Here's how the part is built. I have some questions about the finished solid (model axes, mm). Face numbers are marked on the shaded views. A direction names the side the tool comes from. Round coordinates to 2 decimals unless told otherwise and drop trailing zeros. Loops run counter-clockwise (first coordinate to the right, second up) from the corner with the lowest first, then second, coordinate; pieces in that order, holes last. Notation, with made-up numbers: M 79.5,-4.5 L 131.5,-4.5 A7 cw 131.5,8.5 Z; hole C 86.5,-16.75 d6. An arc over 180 degrees is marked long. Answer as a JSON object with one key per item and string values.
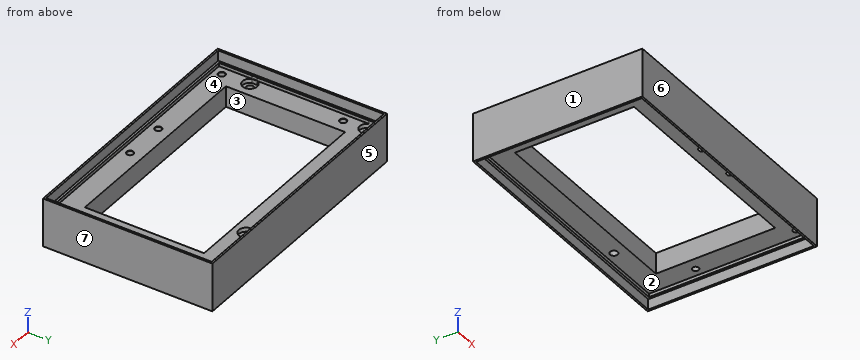
from build123d import *

# Parameters (mm, degrees)
F0_W            = 124.8
F0_H            = 81
F1_DEPTH        = 23.2
F2_W            = 123
F2_H            = 79.2
F3_DEPTH        = 5
F4_W            = 123
F4_H            = 79.2
F5_DEPTH        = 5
F6_W            = 120.8
F6_H            = 77
F7_DEPTH        = 1.6
F8_W            = 120.8
F8_H            = 77
F9_DEPTH        = 1.6
F10_W           = 100.8
F10_H           = 57
F11_DEPTH       = 16.601
F13_R           = 3.5
F14_DEPTH       = 6.601
F15_DEPTH       = 2
F12_R           = 1.8
F16_DEPTH       = 16.601
F17_R           = 1.8
F19_DEPTH       = 16.601
F18_R           = 3.5
F20_DEPTH       = 2
F21_R           = 1.8
F23_DEPTH       = 16.601
F22_R           = 1.8
F24_DEPTH       = 2
F22_R_2         = 3.5
F25_DEPTH       = 25
F27_D           = 3
F27_CSINK_D     = 3.28
F27_CSINK_ANGLE = 90


with BuildPart() as f1:
    # F0 (on Top) → F1 (new body)
    with BuildSketch(Plane.XY):
        Rectangle(F0_W, F0_H)
    extrude(amount=F1_DEPTH)

    # F2 (on face) → F3 (cut)
    with BuildSketch(Plane.XY.offset(23.2)):
        Rectangle(F2_W, F2_H)
    extrude(amount=-F3_DEPTH, mode=Mode.SUBTRACT)

    # F4 (on face) → F5 (cut)
    with BuildSketch(Plane(origin=(0, 0, 0), x_dir=(1, 0, 0), z_dir=(0, 0, -1))):
        Rectangle(F4_W, F4_H)
    extrude(amount=-F5_DEPTH, mode=Mode.SUBTRACT)

    # F6 (on face) → F7 (cut)
    with BuildSketch(Plane.XY.offset(18.2)):
        Rectangle(F6_W, F6_H)
    extrude(amount=-F7_DEPTH, mode=Mode.SUBTRACT)

    # F8 (on face) → F9 (cut)
    with BuildSketch(Plane(origin=(0, 0, 5), x_dir=(1, 0, 0), z_dir=(0, 0, -1))):
        Rectangle(F8_W, F8_H)
    extrude(amount=-F9_DEPTH, mode=Mode.SUBTRACT)

    # F10 (on face) → F11 (cut, through all)
    with BuildSketch(Plane(origin=(0, 0, 6.6), x_dir=(1, 0, 0), z_dir=(0, 0, -1))):
        Rectangle(F10_W, F10_H)
    extrude(amount=-F11_DEPTH, mode=Mode.SUBTRACT)

    # F13 (on face) → F14 (cut, through all)
    with BuildSketch(Plane.XY.offset(16.6)):
        with Locations((-57.1, 34.5)):
            Circle(F13_R)
    extrude(amount=F14_DEPTH, mode=Mode.SUBTRACT)

    # F13 (on face) → F15 (cut)
    with BuildSketch(Plane.XY.offset(16.6)):
        with Locations((-57.1, 34.5)):
            Circle(F13_R)
    extrude(amount=-F15_DEPTH, mode=Mode.SUBTRACT)

    # F12 (on face) → F16 (cut, through all)
    with BuildSketch(Plane.XY.offset(16.6)):
        with Locations((-57.1, 34.5)):
            Circle(F12_R)
    extrude(amount=-F16_DEPTH, mode=Mode.SUBTRACT)

    # F17 (on face) → F19 (cut, through all)
    with BuildSketch(Plane.XY.offset(16.6)):
        with Locations((29.3, 34.5)):
            Circle(F17_R)
    extrude(amount=-F19_DEPTH, mode=Mode.SUBTRACT)

    # F18 (on face) → F20 (cut)
    with BuildSketch(Plane.XY.offset(16.6)):
        with Locations((29.3, 34.5)):
            Circle(F18_R)
    extrude(amount=-F20_DEPTH, mode=Mode.SUBTRACT)

    # F21 (on face) → F23 (cut, through all)
    with BuildSketch(Plane.XY.offset(16.6)):
        with Locations((-57.1, -21.5)):
            Circle(F21_R)
    extrude(amount=-F23_DEPTH, mode=Mode.SUBTRACT)

    # F22 (on face) → F24 (cut)
    with BuildSketch(Plane.XY.offset(16.6)):
        with BuildLine():
            ThreePointArc((-60.4, -22.666190379), (-56.5083920217, -24.9496376621), (-53.6, -21.5))
            ThreePointArc((-53.6, -21.5), (-56.5083920217, -18.0503623379), (-60.4, -20.333809621))
            Line((-60.4, -20.333809621), (-60.4, -22.666190379))
        make_face()
        with Locations((-57.1, -21.5)):
            Circle(F22_R, mode=Mode.SUBTRACT)
    extrude(amount=-F24_DEPTH, mode=Mode.SUBTRACT)

    # F22 (on face) → F25 (cut)
    with BuildSketch(Plane.XY.offset(16.6)):
        with Locations((-57.1, -21.5)):
            Circle(F22_R_2)
    extrude(amount=F25_DEPTH, mode=Mode.SUBTRACT)

    # F27 (through all)
    with Locations(Plane.XY.offset(16.6)):
        with Locations((56.4, 13.5), (56.4, -34.5), (9.1, -34.5), (-11.06, -34.5), (-56.4, -34.5), (-56.4, 23.54)):
            CounterSinkHole(F27_D / 2, F27_CSINK_D / 2, counter_sink_angle=F27_CSINK_ANGLE)


solid = f1.part
Item 1: I want a section at C-C, the plane z = 1.75. Please give me the cut outline in (x, y).
Resolved:
{"outline": "M -62.4,-40.5 L 62.4,-40.5 L 62.4,40.5 L -62.4,40.5 Z; hole M -61.5,-39.6 L 61.5,-39.6 L 61.5,39.6 L -61.5,39.6 Z"}
Item 2: If we mould it in two halves opening along Y, with no side actions, what happens to the marked faces 4, 5, 6 and 7? For each: pulls with the +Y half, pulls with the -Y half, needs draft (parallel to the pull), parting line crosses it, or undercut.
Resolved:
{"face 4": "undercut", "face 5": "pulls with the +Y half", "face 6": "pulls with the -Y half", "face 7": "needs draft"}
Item 3: Please list where these lines run through material, in increasing order: probe 1 along X at (y, z) = (13.5, 14.5); probe 2 along X at (y, z) = (-34.5, 10.5); probe 3 along X at (y, z) = (15.5, 2). Write a range as from..to.
Resolved:
{"probe 1": "-62.4..-50.4, 50.4..54.9, 57.9..62.4", "probe 2": "-62.4..-57.9, -54.9..-12.56, -9.56..7.6, 10.6..54.9, 57.9..62.4", "probe 3": "-62.4..-61.5, 61.5..62.4"}
Item 4: I'm going to push flat-ended pins straight in: pin 1 Ø3.5 at (x, y) = (9.1, -34.5) entering from -Z; pin 2 Ø4 at (x, y) = (-56.4, 23.54) entering from +Z. Where does each tip first touch, or does it pass through?
Resolved:
{"pin 1": "z = 6.6", "pin 2": "z = 16.6"}
Item 5: On a 3-axis mill with a long thin cutter (end or side, diameter ignored), from which of +Z, -Z, +X, -X, +Y, -Y can I reach the whole of each face in a straight line? I mean the marked faces 1, 2 and 3. Say none if no direction works.
Resolved:
{"face 1": "+Z, -Z, -X, +Y, -Y", "face 2": "-Z", "face 3": "+Z, -Z"}
Item 6: I want a section at A-A, the plane x = 9.1. State how many separate pieces and enclosed holes the cut face has, then the cut area to 3 significant figures.
Resolved:
{"separate pieces": "3", "enclosed holes": "0", "area": "241 mm²"}
